Geometry: see drawing. Coordinates: mm, zero at the bounding-box minimum. Round coordinates to 2 decimals unless told otherwise and drop trailing zeros. Order: outer loops, then holes, each group sorted by start corner. A loop starts at its lowest first (then second) coordinate and runs counter-clockwise, first axis right, second up. Notation, with made-up numbers: (35, -26) -> (82, -26) arc R13 cw to (82, -17) -> close; hole circle Ø2 at (89, 36.25). An arc over 180 degrees is marked (long way). Answer as CSV lines item,"result". Start each with the question number.
(1) Line query: line 1 along Z through (x, y) = (2.2, 9); line 2 along Z through (x, y) = (1.2, 3); line 3 along Y through (x, z) = (2.5, 32). Output: solid intervals per line, ascending. Write a range as from..to.
(2) Section query B-B (x = 1.6). Output: boundary loops of the cut face in (y, z).
(3) Contact query for a flat-ended pin moving along its axis: P1, Ø3, axis at y = 9.5, z = 46.5, coming from the -X side. Output: stop coordinate, or through.
(4) Section query C-C (z = 32.5). Output: boundary loops of the cut face in (x, y), plus the area to 3 significant figures.
(5) Section query A-A (y = 11). Output: boundary loops of the cut face in (x, z).
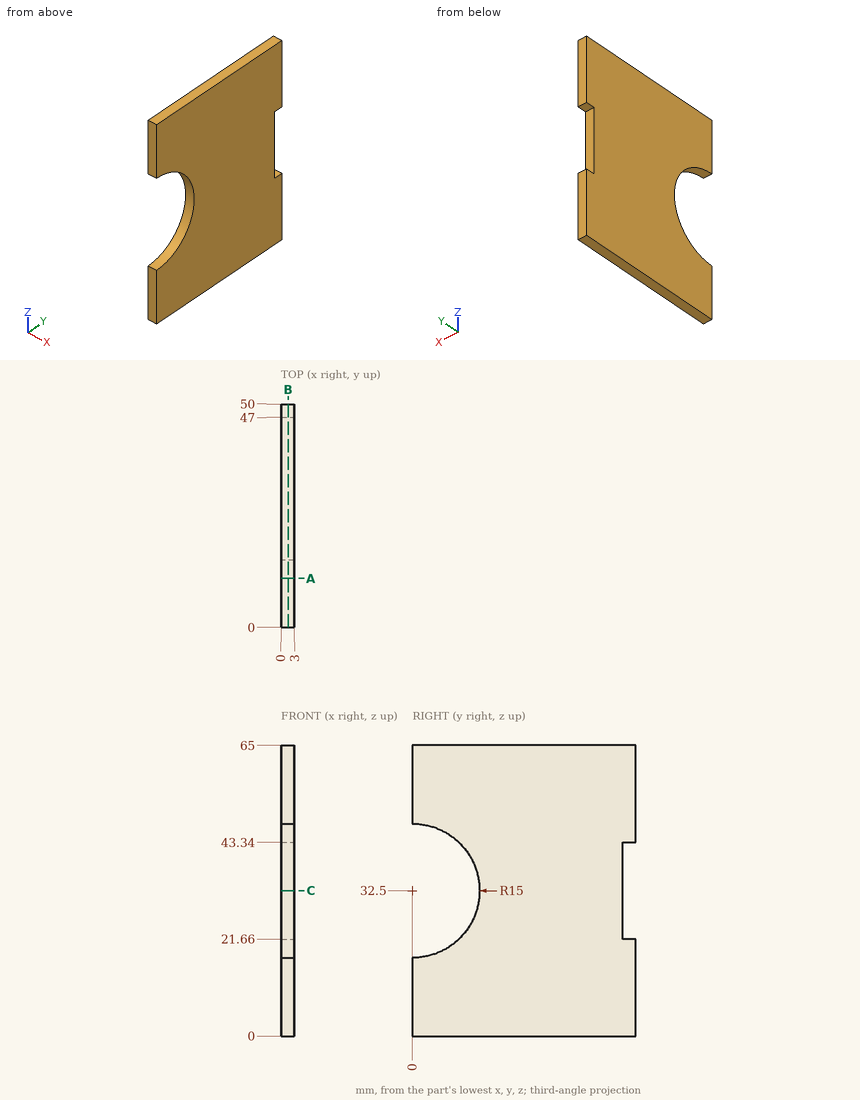
Answer block:
1,line 1,"0..20.5, 44.5..65"
1,line 2,"0..17.8, 47.2..65"
1,line 3,"14.99..47"
2,outline,"(0, 0) -> (50, 0) -> (50, 21.66) -> (47, 21.66) -> (47, 43.34) -> (50, 43.34) -> (50, 65) -> (0, 65) -> (0, 47.5) arc R15 cw to (0, 17.5) -> close"
3,P1,"x = 0"
4,outline,"(0, 15) -> (3, 15) -> (3, 47) -> (0, 47) -> close"
4,area,"96.0 mm2"
5,outline,"(0, 0) -> (3, 0) -> (3, 22.3) -> (0, 22.3) -> close; (0, 42.7) -> (3, 42.7) -> (3, 65) -> (0, 65) -> close"
